from build123d import *

# Parameters (mm, degrees)
EXTRUDE_1_DEPTH     = 20
SKETCH_2_R          = 15
SKETCH_2_R_2        = 10
SKETCH_2_W          = 70
SKETCH_2_H          = 30
CUT_EXTRUDE_2_DEPTH = 20


with BuildPart() as part:
    # 草图1 → 凸台-拉伸1 (new body)
    with BuildSketch(Plane.XY):
        Polygon((-938.635343121, 0), (61.364656879, 0), (61.364656879, 400), (-338.635343121, 360.555127546), align=None)
    extrude(amount=EXTRUDE_1_DEPTH)

    # 草图2 → 切除-拉伸2 (cut)
    with BuildSketch(Plane.XY):
        with Locations(Location((-88.635343121, 150, 0), (0, 0, 180))):
            Circle(SKETCH_2_R)
        with Locations(Location((-638.635343121, 25, 0), (0, 0, 180))):
            Circle(SKETCH_2_R_2)
        with Locations((-193.635343121, 335)):
            Rectangle(SKETCH_2_W, SKETCH_2_H)
        with Locations((6.364656879, 335)):
            Rectangle(SKETCH_2_W, SKETCH_2_H)
    extrude(amount=CUT_EXTRUDE_2_DEPTH, mode=Mode.SUBTRACT)


solid = part.part
Read the model definition and answer for the solid it produces. Units are mm, in the model's axes. A direction names the side the tool comes from. Give positions to 0.01 mm unless a question says otherwise; leave off trailing zeros. Write each loop counter-clockwise with the first axis right and the second up, starting at its lowest first coordinate (ties: lowest second). Pieces come first, ordered by that corner, then holes. Notation, with made-up numbers: (61.25, 85.5) - (92.25, 85.5) arc R16 ccw to (92.25, 107.5) - close; hole circle Ø6 at (-8.5, -38.5). An arc over 180 degrees is marked (long way). Return JSON: item names as keys, results as strings.
Q1. For a pull along X with two mould halves and no side action, classify faces 3 (the face through (-634.44, 182.8, 9.86)), 4 (the face through (6, 350, 10)), 5 (the face through (-446, 0, 10)), 6 (the face through (61.365, 197, 10)) as released by +X, released by -X, zero draft, split by the parting line, or undercut.
Reply:
{"face 3": "released by -X", "face 4": "undercut", "face 5": "zero draft", "face 6": "released by +X"}
Q2. A cutting plane is placed at C-C, the plane y = 332. Determine the outline of the cut face in (x, z).
Reply:
{"outline": "(-386.15, 0) - (-228.64, 0) - (-228.64, 20) - (-386.15, 20) - close; (-158.64, 0) - (-28.64, 0) - (-28.64, 20) - (-158.64, 20) - close; (41.36, 0) - (61.36, 0) - (61.36, 20) - (41.36, 20) - close"}
Q3. Given P1, Ø2, axis at x = -194, z = 17.5, coming from the +Y side; P2, Ø2, axis at x = -509, z = 13.5, coming from the +Y side; P3, Ø6, axis at x = -176.5, z = 11, coming from the +Y side; P4, Ø18, axis at x = -638.64, y = 25, coming from the -Z side, each flat-ended and moving along its own axis, determine where each tip first touches the part or whether it passes through.
Reply:
{"P1": "y = 374.92", "P2": "y = 258.78", "P3": "y = 376.84", "P4": "through"}
Q4. For faces 1 (the face through (-228.635, 335, 10)), 2 (the face through (-335, 158, 0)), determine the directions among +Z, -Z, +X, -X, +Y, -Y from which every point of the face is accessible in a straight line to the end or side of a thin tool.
Reply:
{"face 1": "+Z, -Z", "face 2": "-Z, +X, -X, +Y, -Y"}
Q5. Consider line 1 along X through (y, z) = (325.5, 10.25); line 2 along Y through (x, z) = (-203, 9.5); line 3 along X through (y, z) = (150, 4.5). Determine where each line is inside the solid, lowest interval first. Write a range as [from, to].
Reply:
{"line 1": "[-396.97, -228.64], [-158.64, -28.64], [41.36, 61.36]", "line 2": "[0, 320], [350, 373.93]", "line 3": "[-689.02, -103.64], [-73.64, 61.36]"}
Q6. A cutting plane is placed at B-B, the plane y = 150. Determine the outline of the cut face in (x, z), and give its area (3 significant figures).
Reply:
{"outline": "(-689.02, 0) - (-103.64, 0) - (-103.64, 20) - (-689.02, 20) - close; (-73.64, 0) - (61.36, 0) - (61.36, 20) - (-73.64, 20) - close", "area": "14,400 mm²"}
Q7. A cutting plane is placed at D-D, the plane y = 25. Determine the outline of the cut face in (x, z).
Reply:
{"outline": "(-897.03, 0) - (-648.64, 0) - (-648.64, 20) - (-897.03, 20) - close; (-628.64, 0) - (61.36, 0) - (61.36, 20) - (-628.64, 20) - close"}
Q8. A cutting plane is placed at A-A, the plane z = 10.5. Determine the outline of the cut face in (x, y).
Reply:
{"outline": "(-938.64, 0) - (61.36, 0) - (61.36, 400) - (-338.64, 360.56) - close; hole circle Ø20 at (-638.64, 25); hole (-228.64, 320) - (-158.64, 320) - (-158.64, 350) - (-228.64, 350) - close; hole circle Ø30 at (-88.64, 150); hole (-28.64, 320) - (41.36, 320) - (41.36, 350) - (-28.64, 350) - close"}
